from build123d import *

# Parameters (mm, degrees)
SKETCH1_W           = 165.1
SKETCH1_H           = 25.4
BOSS_EXTRUDE1_DEPTH = 6.35
FILLET1_R           = 1.27
SKETCH2_R           = 3.175
SKETCH2_R_2         = 6.35
CUT_EXTRUDE1_DEPTH  = 84.762252835
SKETCH3_R           = 9.525
CUT_EXTRUDE2_DEPTH  = 3.571875
CUT_EXTRUDE3_DEPTH  = 84.762252835
SKETCH5_R           = 3.175
CUT_EXTRUDE4_DEPTH  = 84.762252956


with BuildPart() as part:
    # Sketch1 → Boss-Extrude1 (new body)
    with BuildSketch(Plane(origin=(0, 0, 0), x_dir=(1, 0, 0), z_dir=(0, 1, 0))):
        Rectangle(SKETCH1_W, SKETCH1_H)
    extrude(amount=BOSS_EXTRUDE1_DEPTH)

    # Fillet1
    fillet1_edges = [part.edges().sort_by_distance(p)[0] for p in [
        (0, 6.35, -12.7),
        (0, 0, -12.7),
        (0, 0, 12.7),
        (0, 6.35, 12.7),
    ]]
    fillet(fillet1_edges, radius=FILLET1_R)

    # Sketch2 → Cut-Extrude1 (cut, through all)
    with BuildSketch(Plane(origin=(0, 6.35, 0), x_dir=(1, 0, 0), z_dir=(0, 1, 0))):
        with Locations(Location((-69.85, 0, 0), (0, 0, 270))):
            Circle(SKETCH2_R)
        with Locations(Location((69.85, 0, 0), (0, 0, 270))):
            Circle(SKETCH2_R_2)
        with Locations(Location((-44.45, 0, 0), (0, 0, 270))):
            Circle(SKETCH2_R)
    extrude(amount=-CUT_EXTRUDE1_DEPTH, mode=Mode.SUBTRACT)

    # Sketch3 → Cut-Extrude2 (cut)
    with BuildSketch(Plane.XZ):
        with Locations(Location((69.85, 0, 0), (0, 0, 270))):
            Circle(SKETCH3_R)
    extrude(amount=-CUT_EXTRUDE2_DEPTH, mode=Mode.SUBTRACT)

    # Sketch4 → Cut-Extrude3 (cut, through all)
    with BuildSketch(Plane.XZ):
        with BuildLine():
            Line((75.385801658, 11.43), (82.55, 11.43))
            Line((82.55, 11.43), (82.55, 12.7))
            Line((82.55, 12.7), (69.85, 12.7))
            ThreePointArc((69.85, 12.7), (72.689806331, 12.378428818), (75.385801658, 11.43))
        make_face()
        with BuildLine():
            ThreePointArc((75.385801658, 11.43), (80.610917272, 6.744824643), (82.55, 0))
            Line((82.55, 0), (82.55, 11.43))
            Line((82.55, 11.43), (75.385801658, 11.43))
        make_face()
        with BuildLine():
            ThreePointArc((82.55, 0), (80.610917272, -6.744824643), (75.385801658, -11.43))
            Line((75.385801658, -11.43), (82.55, -11.43))
            Line((82.55, -11.43), (82.55, 0))
        make_face()
        with BuildLine():
            ThreePointArc((75.385801658, -11.43), (72.689806331, -12.378428818), (69.85, -12.7))
            Line((69.85, -12.7), (82.55, -12.7))
            Line((82.55, -12.7), (82.55, -11.43))
            Line((82.55, -11.43), (75.385801658, -11.43))
        make_face()
    extrude(amount=-CUT_EXTRUDE3_DEPTH, mode=Mode.SUBTRACT)

    # Sketch5 → Cut-Extrude4 (cut, through all)
    with BuildSketch(Plane.XZ):
        with Locations(Location((50.8, 0, 0), (0, 0, 270))):
            Circle(SKETCH5_R)
        with Locations(Location((38.1, 0, 0), (0, 0, 270))):
            Circle(SKETCH5_R)
    extrude(amount=-CUT_EXTRUDE4_DEPTH, mode=Mode.SUBTRACT)

    # Sketch8 → Cut-Revolve1 (revolve, cut)
    with BuildSketch(Plane.XY, mode=Mode.PRIVATE) as cut_revolve1_sk:
        Polygon((77.91821119, 6.35), (76.2, 6.35), (76.2, 3.571875), (76.681310248, 3.571875), align=None)
    revolve(cut_revolve1_sk.sketch.rotate(Axis((69.85, 3.571875, 0), (0, 1, 0)), 90), axis=Axis((69.85, 3.571875, 0), (0, 1, 0)), mode=Mode.SUBTRACT)


solid = part.part
Work out the finished part from the listing and answer in its coordinate system (mm). A direction names the side the tool comes from. Give positions to 0.01 mm unless a question says otherwise; leave off trailing zeros. Write each loop counter-clockwise with the first axis right and the second up, starting at its lowest first coordinate (ties: lowest second). Pieces come first, ordered by that corner, then holes. Notation, with made-up numbers: M 37,26 L 49,26 A9 ccw 49,38 Z; hole C 58.5,16 d2. An arc over 180 degrees is marked long. Answer as CSV lines item,"result".
Q1. Find the intervals of material crossed by probe 1 along X at (y, z) = (0.5, -2.75); probe 2 along X at (y, z) = (1.75, -0.5); probe 3 along X at (y, z) = (1.25, 3.5), in increasing order. Write a range as [from, to].
A:
probe 1,"x = [-82.55, -71.44], [-68.26, -46.04], [-42.86, 36.51], [39.69, 49.21], [52.39, 60.73], [78.97, 82.25]"
probe 2,"x = [-82.55, -72.99], [-66.71, -47.59], [-41.31, 34.96], [41.24, 47.66], [53.94, 60.34], [79.36, 82.54]"
probe 3,"x = [-82.55, 60.99], [78.71, 82.06]"
Q2. A cutting plane is placed at A-A on x = 50.8. Write down the section's boundary in (y, z) (3 decimals).
A:
outline,"M 0,-11.43 A1.27 ccw 1.27,-12.7 L 5.08,-12.7 A1.27 ccw 6.35,-11.43 L 6.35,-3.175 L 0,-3.175 Z; M 0,3.175 L 6.35,3.175 L 6.35,11.43 A1.27 ccw 5.08,12.7 L 1.27,12.7 A1.27 ccw 0,11.43 Z"
Q3. The mould has two halves that part along X. Classify faces 1 (the flat face through (-7, 3, -12.7)), 2 (the cylindrical face through (35, 3.13, 0.69)), 3 (the cylindrical face through (79.3, 1.8, 1.2)), 4 (the flat face through (-82.55, 3, 0)): +X half, -X half, draft (parallel to the pull), parting line (faces both ways), or undercut.
A:
face 1,"draft"
face 2,"undercut"
face 3,"undercut"
face 4,"-X half"
Q4. A cutting plane is placed at B-B on y = 2.5. Write down the section's boundary in (x, z) (3 decimals), plus the area to 3 significant figures.
A:
outline,"M -82.55,-12.7 L 69.85,-12.7 A12.7 ccw 69.85,12.7 L -82.55,12.7 Z; hole C -69.85,0 d6.35; hole C -44.45,0 d6.35; hole C 38.1,0 d6.35; hole C 50.8,0 d6.35; hole C 69.85,0 d19.05"
area,"3,710 mm²"
Q5. A tool of negligible diameter and unlimited length cuts with its end or side. For faces 5 (the conical face through (65.181, 3.746, 5.092)), 6 (the flat face through (64, 3.572, -4)), from which of +Z, -Z, +X, -X, +Y, -Y can it reach the whole face along a straight path? Write none if from no direction.
A:
face 5,"+Y"
face 6,"-Y"
